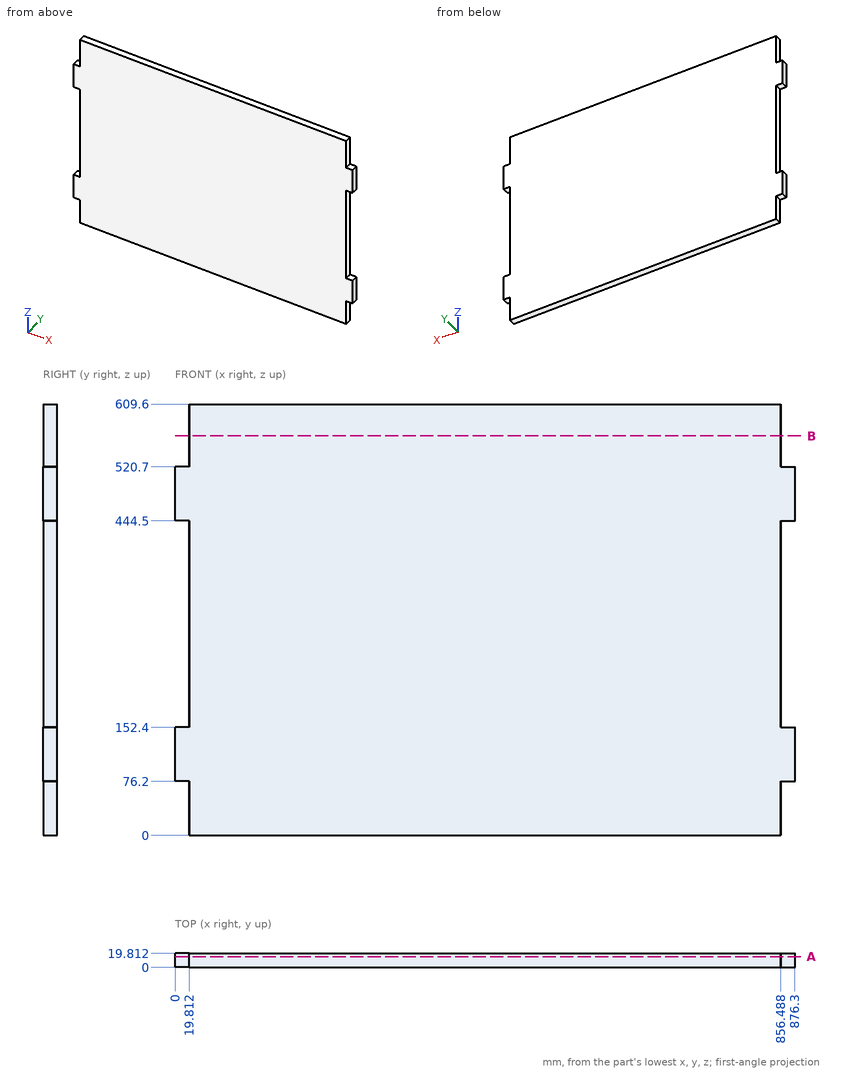
Verification items for this drawing (mm, ordinates from the low corner). Round coordinates to 2 decimals unless told otherwise and drop trailing zeros. Write each loop counter-clockwise with the first axis right and the second up, starting at its lowest first coordinate (ties: lowest second). Pieces come first, ordered by that corner, then holes. Notation, with made-up numbers: M 61,8.25 L 69,8.25 A18 cw 69,15.25 Z; hole C -20.75,54.5 d5. An arc over 180 degrees is marked long. Write item = value, one per line. Start each with the question number.
1. Gauge pin test, flat ends, axial feed: pin 1 (6 mm diameter, centred on x = 871, y = 8.5, fed in from +Z); pin 2 (10 mm diameter, centred on x = 6.5, y = 5.5, fed in from -Z); pin 3 (4 mm diameter, centred on y = 13.5, z = 273, fed in from +X); pin 4 (10 mm diameter, centred on x = 283, z = 279.5, fed in from -Y). Record the tip position at first contact, or that the pin passes through.
2. Section check A-A, the plane y = 15.25. Record the cut outline in (x, z).
3. Scan line: line 1 (X direction, y = 9.75, z = 545). Record every from-to range of solid material in increasing order. Write a range as [from, to].
4. Section check B-B, the plane z = 564.5. Record the cut outline in (x, y).
Results found:
q1.pin_1 = 520.7
q1.pin_2 = 76.2
q1.pin_3 = 856.49
q1.pin_4 = 0
q2.outline = M 0,76.2 L 19.81,76.2 L 19.81,0 L 856.49,0 L 856.49,76.2 L 876.3,76.2 L 876.3,152.4 L 856.49,152.4 L 856.49,444.5 L 876.3,444.5 L 876.3,520.7 L 856.49,520.7 L 856.49,609.6 L 19.81,609.6 L 19.81,520.7 L 0,520.7 L 0,444.5 L 19.81,444.5 L 19.81,152.4 L 0,152.4 Z
q3.line_1 = [19.81, 856.49]
q4.outline = M 19.81,0 L 856.49,0 L 856.49,19.81 L 19.81,19.81 Z
